Geometry check sheet. Reference: the model listing, model coordinates, mm. A direction names the side the tool comes from. Give positions to 0.01 mm unless a question says otherwise; leave off trailing zeros. Write each loop counter-clockwise with the first axis right and the second up, starting at its lowest first coordinate (ties: lowest second). Pieces come first, ordered by that corner, then holes. Notation, with made-up numbers: (50.25, 74.5) -> (92.25, 74.5) arc R19 cw to (92.25, 88.5) -> close; hole circle Ø6 at (48, 0). An arc over 180 degrees is marked (long way). Use a Markdown table: item, result. Add a question column.
from build123d import *

# Parameters (mm, degrees)
F1_DEPTH = 5


with BuildPart() as f1:
    # F0 (on Top) → F1 (new body)
    with BuildSketch(Plane.XY):
        with BuildLine():
            Line((21.641407, 3.508914), (21.122372, 25.04304))
            Line((21.122372, 25.04304), (-28.877628, 25.04304))
            Line((-28.877628, 25.04304), (-28.877628, 3.54304))
            ThreePointArc((-28.877628, 3.54304), (-28.438288, 2.48238), (-27.377628, 2.04304))
            Line((-27.377628, 2.04304), (-26.754604, 2.04304))
            ThreePointArc((-26.754604, 2.04304), (-26.075812, 2.205415), (-25.543978, 2.657385))
            ThreePointArc((-25.543978, 2.657385), (-21.957112, 4.279539), (-18.717504, 2.04304))
            ThreePointArc((-18.717504, 2.04304), (-18.326309, 0.003702), (-19.010222, -1.95696))
            ThreePointArc((-19.010222, -1.95696), (-22.01054, -3.692708), (-25.239965, -2.433524))
            ThreePointArc((-25.239965, -2.433524), (-25.738738, -2.08125), (-26.336586, -1.95696))
            Line((-26.336586, -1.95696), (-27.377628, -1.95696))
            ThreePointArc((-27.377628, -1.95696), (-28.438288, -2.3963), (-28.877628, -3.45696))
            Line((-28.877628, -3.45696), (-28.877628, -24.95696))
            Line((-28.877628, -24.95696), (21.122372, -24.95696))
            Line((21.122372, -24.95696), (21.122372, -3.45696))
            ThreePointArc((21.122372, -3.45696), (21.561712, -2.3963), (22.622372, -1.95696))
            Line((22.622372, -1.95696), (24.022886, -1.95696))
            ThreePointArc((24.022886, -1.95696), (24.637921, -2.088847), (25.144802, -2.461317))
            ThreePointArc((25.144802, -2.461317), (28.452575, -3.793768), (31.509193, -1.95696))
            ThreePointArc((31.509193, -1.95696), (30.43203, 3.469536), (24.963791, 2.629592))
            ThreePointArc((24.963791, 2.629592), (24.435111, 2.19659), (23.769215, 2.043048))
            Line((23.769215, 2.043048), (23.136191, 2.045066))
            ThreePointArc((23.136191, 2.045066), (22.091459, 2.473366), (21.641407, 3.508914))
        make_face()
    extrude(amount=F1_DEPTH)


solid = f1.part
1) Sectioned sample at B-B, the plane y = -15.5. Enter the section's corners in (x, z), and give its area (3 significant figures).
2) Sectioned sample at A-A, the plane z = 3.65. Enter the section's corners in (x, y), and give its area (3 significant figures).
3) Tool access check on faces 1 (the face through (21.55, -2.41, 2.46)), 2 (the face through (-26.085, 2.201, 2.465)), 3 (the face through (24.44, 2.2, 2.46)), 4 (the face through (-28.45, 2.494, 2.465)). Record the directions out of +Z, -Z, +X, -X, +Y, -Y that give a thin tool (end or side, any length) a straight path to the whole face; none if there is none.
4) Sectioned sample at C-C, the plane y = -0.5. Enter the section's corners in (x, z).
5) Material ranges on probe 1 along X at (y, z) = (-15.5, 1.35); probe 2 along X at (y, z) = (3.5, 4.3); probe 3 along Y at (x, z) = (-20.5, 0.35), recorded low to high. Write a range as [from, to].
6) Gauge pin test, flat ends, axial feed: P1, Ø2.5, axis at y = -19, z = 2, coming from the +X side; P2, Ø1.5, axis at x = 23.5, z = 3.5, coming from the -Y side; P3, Ø2, axis at y = 7, z = 1, coming from the +X side. Record the tip position at first contact, or that the pin passes through.
Check values:
| question | item | result |
|---|---|---|
| 1 | outline | (-28.88, 0) -> (21.12, 0) -> (21.12, 5) -> (-28.88, 5) -> close |
| 1 | area | 250 mm² |
| 2 | outline | (-28.88, -24.96) -> (21.12, -24.96) -> (21.12, -3.46) arc R1.5 cw to (22.62, -1.96) -> (24.02, -1.96) arc R1.5 cw to (25.14, -2.46) arc R4 ccw (long way) to (24.96, 2.63) arc R1.5 cw to (23.77, 2.04) -> (23.14, 2.05) arc R1.5 cw to (21.64, 3.51) -> (21.12, 25.04) -> (-28.88, 25.04) -> (-28.88, 3.54) arc R1.5 ccw to (-27.38, 2.04) -> (-26.75, 2.04) arc R1.5 ccw to (-25.54, 2.66) arc R4 cw to (-18.72, 2.04) arc R4 cw to (-19.01, -1.96) arc R4 cw to (-25.24, -2.43) arc R1.5 ccw to (-26.34, -1.96) -> (-27.38, -1.96) arc R1.5 ccw to (-28.88, -3.46) -> close |
| 2 | area | 2,510 mm² |
| 3 | face 1 | +Z, -Z, -Y |
| 3 | face 2 | +Z, -Z |
| 3 | face 3 | +Z, -Z, +Y |
| 3 | face 4 | +Z, -Z, -X |
| 4 | outline | (-18.4, 0) -> (32.08, 0) -> (32.08, 5) -> (-18.4, 5) -> close |
| 5 | probe 1 | [-28.88, 21.12] |
| 5 | probe 2 | [-28.88, -24.71], [-19.92, 21.64], [25.89, 30.39] |
| 5 | probe 3 | [-24.96, -3.27], [3.86, 25.04] |
| 6 | P1 | x = 21.12 |
| 6 | P2 | y = -1.97 |
| 6 | P3 | x = 21.58 |
